```python
from build123d import *

# Parameters (mm, degrees)
F0_W     = 31.75
F0_H     = 31.75
F1_DEPTH = 31.75
F2_W     = 31.75
F2_H     = 31.75
F3_DEPTH = 79.375
F4_DEPTH = 60.325
F5_DEPTH = 41.275


with BuildPart() as f1:
    # F0 (on Top) → F1 (new body)
    with BuildSketch(Plane.XY):
        Polygon((-69.85, 44.45), (-69.85, 76.2), (-127, 76.2), (-127, 25.4), (-85.725, 25.4), (-85.725, -25.4), (-127, -25.4), (-127, -76.2), (-69.85, -76.2), (-69.85, -44.45), (-69.85, -25.4), (-69.85, 25.4), align=None)
        Polygon((127, 25.4), (127, 76.2), (69.85, 76.2), (69.85, 44.45), (69.85, 25.4), (69.85, -25.4), (69.85, -44.45), (69.85, -76.2), (127, -76.2), (127, -25.4), (85.725, -25.4), (85.725, 25.4), align=None)
        Polygon((-38.1, -44.45), (-38.1, 44.45), (-69.85, 44.45), (-69.85, 25.4), (-69.85, -25.4), (-69.85, -44.45), align=None)
        with Locations((-53.975, 60.325)):
            Rectangle(F0_W, F0_H)
        with Locations((-53.975, -60.325)):
            Rectangle(F0_W, F0_H)
        with BuildLine():
            Line((0, 15.875), (0, 76.2))
            Line((0, 76.2), (-38.1, 76.2))
            Line((-38.1, 76.2), (-38.1, 44.45))
            Line((-38.1, 44.45), (-38.1, -44.45))
            Line((-38.1, -44.45), (-38.1, -76.2))
            Line((-38.1, -76.2), (0, -76.2))
            Line((0, -76.2), (0, -15.875))
            ThreePointArc((0, -15.875), (-15.875, 0), (0, 15.875))
        make_face()
        with BuildLine():
            Line((38.1, 44.45), (38.1, 76.2))
            Line((38.1, 76.2), (0, 76.2))
            Line((0, 76.2), (0, 15.875))
            ThreePointArc((0, 15.875), (11.2253201513, 11.2253201513), (15.875, 0))
            ThreePointArc((15.875, 0), (11.2253201513, -11.2253201513), (0, -15.875))
            Line((0, -15.875), (0, -76.2))
            Line((0, -76.2), (38.1, -76.2))
            Line((38.1, -76.2), (38.1, -44.45))
            Line((38.1, -44.45), (38.1, 44.45))
        make_face()
        with Locations((53.975, -60.325)):
            Rectangle(F0_W, F0_H)
        Polygon((69.85, 25.4), (69.85, 44.45), (38.1, 44.45), (38.1, -44.45), (69.85, -44.45), (69.85, -25.4), align=None)
        with Locations((53.975, 60.325)):
            Rectangle(F0_W, F0_H)
    extrude(amount=F1_DEPTH)

    # F2 (on face) → F3 (join)
    with BuildSketch(Plane.XY.offset(31.75)):
        with Locations((-53.975, -60.325)):
            Rectangle(F2_W, F2_H)
        with Locations((53.975, -60.325)):
            Rectangle(F2_W, F2_H)
        with Locations((53.975, 60.325)):
            Rectangle(F2_W, F2_H)
        with Locations((-53.975, 60.325)):
            Rectangle(F2_W, F2_H)
    extrude(amount=F3_DEPTH)

    # F2 (on face) → F4 (join)
    with BuildSketch(Plane.XY.offset(31.75)):
        Polygon((-38.1, -44.45), (-38.1, 44.45), (-69.85, 44.45), (-69.85, 25.4), (-69.85, -25.4), (-69.85, -44.45), align=None)
        Polygon((69.85, 25.4), (69.85, 44.45), (38.1, 44.45), (38.1, -44.45), (69.85, -44.45), (69.85, -25.4), align=None)
    extrude(amount=F4_DEPTH)

    # F5 (add): a face of the model
    f5_faces = [f1.faces().sort_by_distance(p)[0] for p in [
        (-36.3961162011, 0, 31.75),
    ]]
    extrude(f5_faces, amount=F5_DEPTH)


solid = f1.part
```
Input: part model. Units: mm. Frame: model coordinates. A direction names the side the tool comes from. Give positions to 0.01 mm unless a question says otherwise; leave off trailing zeros. Loops run counter-clockwise (first coordinate to the right, second up) from the corner with the lowest first, then second, coordinate; pieces in that order, holes last.
1) Section query C-C on x = 0. Return the cut outline in (y, z) (3 decimals), and give its area (3 significant figures).
A:
outline: (-76.2, 0) - (-15.875, 0) - (-15.875, 73.025) - (-76.2, 73.025) - close; (15.875, 0) - (76.2, 0) - (76.2, 73.025) - (15.875, 73.025) - close
area: 8,810 mm2
2) Mould query, pull axis X, two halves, no side actions, for faces 1 (the flat face through (-127, -50, 16)), 2 (the flat face through (69.85, -1, 71)), 3 (the flat face through (-2, -76.2, 42)), 4 (the cylindrical face through (0.7, -15.86, 36)). Classes: released by +X, released by -X, zero draft, split by the parting line, or undercut.
A:
face 1: released by -X
face 2: released by +X
face 3: zero draft
face 4: undercut
3) Reachability of faces 5 (the flat face through (106, 25.4, 16)), 6 (the flat face through (-80, 1, 31.75)), 7 (the flat face through (54, 44.45, 101)) from +Z, -Z, +X, -X, +Y, -Y: full face, straight path, thin tool, end or side. Return the list, or none.
A:
face 5: +Z, -Z, +X
face 6: +Z, -X, +Y, -Y
face 7: +Z, +X, -X
4) Section query B-B on z = 97.5. Return the cut outline in (x, y).
A:
outline: (-69.85, -76.2) - (-38.1, -76.2) - (-38.1, -44.45) - (-69.85, -44.45) - close; (-69.85, 44.45) - (-38.1, 44.45) - (-38.1, 76.2) - (-69.85, 76.2) - close; (38.1, -76.2) - (69.85, -76.2) - (69.85, -44.45) - (38.1, -44.45) - close; (38.1, 44.45) - (69.85, 44.45) - (69.85, 76.2) - (38.1, 76.2) - close
5) Section query A-A on y = 0. Return the cut outline in (x, z) (3 decimals).
A:
outline: (-85.725, 0) - (-15.875, 0) - (-15.875, 73.025) - (-38.1, 73.025) - (-38.1, 92.075) - (-69.85, 92.075) - (-69.85, 31.75) - (-85.725, 31.75) - close; (15.875, 0) - (85.725, 0) - (85.725, 31.75) - (69.85, 31.75) - (69.85, 92.075) - (38.1, 92.075) - (38.1, 73.025) - (15.875, 73.025) - close
6) Section query D-D on z = 20.5. Return the cut outline in (x, y) (3 decimals), and give its area (3 significant figures).
A:
outline: (-127, -76.2) - (127, -76.2) - (127, -25.4) - (85.725, -25.4) - (85.725, 25.4) - (127, 25.4) - (127, 76.2) - (-127, 76.2) - (-127, 25.4) - (-85.725, 25.4) - (-85.725, -25.4) - (-127, -25.4) - close; hole circle Ø31.75 at (0, 0)
area: 33,700 mm2
7) Line query: L1, parallel to Y at x = 0, z = 58.5 (3 decimals); L2, parallel to Y at x = -102, z = 16; L3, parallel to X at y = 51, z = 94.5. Output: solid intervals per line, ascending.
A:
L1: y = -76.2 to -15.875, 15.875 to 76.2
L2: y = -76.2 to -25.4, 25.4 to 76.2
L3: x = -69.85 to -38.1, 38.1 to 69.85
8) Contact query for flat-ended pins moving along their axis: pin 1 (4 mm diameter, centred on x = 73, y = -5.5, fed in from +Z); pin 2 (5 mm diameter, centred on y = -28, z = 72, fed in from -X); pin 3 (10 mm diameter, centred on y = 47.5, z = 67.5, fed in from +X). Output: stop coordinate, or through.
A:
pin 1: stops at z = 31.75
pin 2: stops at x = -69.85
pin 3: stops at x = 69.85
